Drawing for the job (mm, zero at the part's lowest x, y, z). Give positions to 0.01 mm unless a question says otherwise; leave off trailing zeros. Loops run counter-clockwise (first coordinate to the right, second up) from the corner with the lowest first, then second, coordinate; pieces in that order, holes last. Notation, with made-up numbers: (55, 67) -> (108, 67) arc R26 cw to (108, 94) -> close; hole circle Ø9 at (49, 87.25). An arc over 180 degrees is marked (long way). Write item = value, one per line.
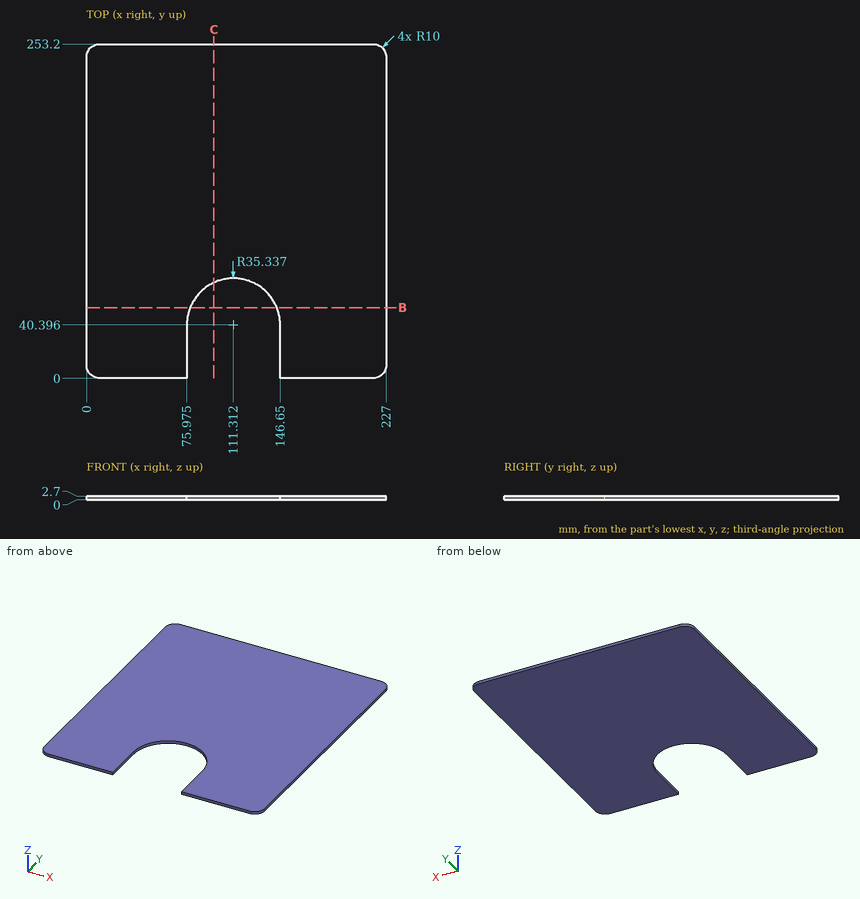
1) Slice it at C-C, the plane x = 96.5. List the corners of the cut face in (y, z).
Resolved:
outline = (72.48, 0) -> (253.2, 0) -> (253.2, 2.7) -> (72.48, 2.7) -> close
2) Slice it at B-B, the plane y = 53.5. List the corners of the cut face in (x, z) (1 decimal).
Resolved:
outline = (0, 0) -> (78.5, 0) -> (78.5, 2.7) -> (0, 2.7) -> close; (144.1, 0) -> (227, 0) -> (227, 2.7) -> (144.1, 2.7) -> close
3) Drop a flat-ended pin along its axis: P1, Ø0.8, axis at y = 23.5, z = 1.5, coming from the -X side. Give the stop position or say it passes through.
Resolved:
P1 = 0
4) Drill centre lines: line 1 along X through (y, z) = (55, 2) (1 decimal); line 2 along Y through (x, z) = (122, 0.3); line 3 along Y through (x, z) = (134, 0.2). Where is each one in solid material? Low to high. Write a range as [from, to].
Resolved:
line_1 = [0, 79.1], [143.5, 227]
line_2 = [74.08, 253.2]
line_3 = [67.49, 253.2]
